Autodesk Inventor part; units mm, degrees
ref_plane "Work Plane1" through (-19.345, 0, 60) normal (1, 0, 0) x (0, 1, 0)
ref_plane "Work Plane2" through (-19.095, 0, 60) normal (1, 0, 0) x (0, 1, 0)
ref_plane "YZ Plane" through (0, 0, 0) normal (1, 0, 0) x (0, 1, 0)
sketch "Sketch1" plane through (0, 0, 0) normal (0, 0, 1) x (1, 0, 0)
  circle A0 centre (0, 0) radius 20
  dimension "d0" = 40
extrude "Extrusion1" add sketch "Sketch1" along normal blind 60
sketch "Sketch2" plane through (0, 0, 60) normal (0, 0, 1) x (1, 0, 0)
  circle A0 centre (0, 0) radius 20
  circle A1 centre (0, 0) radius 19.345
extrude "Extrusion2" add sketch "Sketch2" along normal blind 6.6 contours A1
sketch "Sketch3" plane through (0, 0, 66.6) normal (0, 0, 1) x (1, 0, 0)
  circle A0 centre (0, 0) radius 19.345
  circle A1 centre (0, 0) radius 20
  dimension "d5" = 40
extrude "Extrusion3" add sketch "Sketch3" along normal blind 38 contours A0 | A1
sketch "Sketch4" plane through (0, 0, 104.6) normal (0, 0, 1) x (1, 0, 0)
  circle A0 centre (0, 0) radius 20
  circle A1 centre (0, 0) radius 8
  dimension "d8" = 16
extrude "Extrusion4" add sketch "Sketch4" along normal blind 4 contours A1
sketch "Sketch5" plane through (0, 0, 108.6) normal (0, 0, 1) x (1, 0, 0)
  circle A0 centre (0, 0) radius 8
  line L0 (3.75, 2.9155) -> (3.75, -2.9155)
  line L1 (-3.75, -2.9155) -> (-3.75, 2.9155)
  arc A1 (-3.75, -2.9155) -> (3.75, -2.9155) centre (0, 0) ccw
  arc A2 (3.75, 2.9155) -> (-3.75, 2.9155) centre (0, 0) ccw
  point P0 (-3.75, 0)
  point P1 (0, 5.9024)
  dimension "d13" = 4.75
  dimension "d14" = 4.75
  dimension "d15" = 7.5
  dimension "d16" = 3.75
  dimension "d17" = 7.5
  dimension "d18" = 5.9024
extrude "Extrusion5" add sketch "Sketch5" along normal blind 14 contours L0 A1 L1 A2
sketch "Sketch6" plane through (0, 0, 122.6) normal (0, 0, 1) x (1, 0, 0)
  line L0 (3.75, 2.9155) -> (3.75, -2.9155)
  arc A0 (3.75, 2.9155) -> (-3.75, 2.9155) centre (0, 0) ccw
  line L1 (-3.75, -2.9155) -> (-3.75, 2.9155)
  arc A1 (-3.75, -2.9155) -> (3.75, -2.9155) centre (0, 0) ccw
  circle A2 centre (0, 0) radius 3.25
  dimension "d21" = 6.5
extrude "Extrusion6" add sketch "Sketch6" along normal blind 10 contours A2
chamfer "Chamfer1" distance 1 angle 45 1 edges at (-3.25, 0, 132.6)
chamfer "Chamfer2" distance 1 angle 80 1 edges at (-20, 0, 0) measured on face at (-2.364, 6.2334, 0)
ref_plane "Work Plane1" through (-19.345, 0, 60) normal (1, 0, 0) x (0, 1, 0)
ref_plane "Work Plane2" through (-19.095, 0, 60) normal (1, 0, 0) x (0, 1, 0)
sketch "Sketch8" plane through (-19.095, 0, 60) normal (1, 0, 0) x (0, 1, 0)
  circle A0 centre (0.0498, -2.6078) radius 0.75
  circle A1 centre (0, 4.3902) radius 0.75
  dimension "d31" = 1.5
  dimension "d32" = 1.5
extrude "Extrusion7" add sketch "Sketch8" against normal blind 10
sketch "Sketch9" plane through (0, 0, 104.6) normal (0, 0, 1) x (1, 0, 0)
  circle A0 centre (0, 0) radius 8
  circle A1 centre (0, 0) radius 20
  line L0 (-9, 9) -> (9, 9)
  line L1 (9, 9) -> (9, -9)
  line L2 (9, -9) -> (-9, -9)
  line L3 (-9, -9) -> (-9, 9)
  point P0 (0, 9)
  point P1 (-9, 0)
  dimension "d35" = 18
  dimension "d36" = 18
hole "Hole1" at (-9, 9, 104.6) at (9, 9, 104.6) at (9, -9, 104.6) at (-9, -9, 104.6) direction (0, 0, -1) diameter 2.487 depth 8 tip angle 118
equation "\"d32\" = d31"
equation "\"d36\" = d35"
properties part number "409A587"
Geometry check sheet. Reference: the model listing, model coordinates, mm. A direction names the side the tool comes from. Give positions to 0.01 mm unless a question says otherwise; leave off trailing zeros. Order: outer loops, then holes, each group sorted by start corner. A loop starts at its lowest first (then second) coordinate and runs counter-clockwise, first axis right, second up.
1. Sectioned sample at C-C (z = 33.5). Record the boundary of the cut face in (x, y).
Completed:
outline: circle Ø40 at (0, 0)
2. Sectioned sample at A-A (x = 0). Record the boundary of the cut face in (y, z) (3 decimals).
Completed:
outline: (-20, 5.671) - (-19, 0) - (19, 0) - (20, 5.671) - (20, 60) - (19.345, 60) - (19.345, 66.6) - (20, 66.6) - (20, 104.6) - (8, 104.6) - (8, 108.6) - (4.75, 108.6) - (4.75, 122.6) - (3.25, 122.6) - (3.25, 131.6) - (2.25, 132.6) - (-2.25, 132.6) - (-3.25, 131.6) - (-3.25, 122.6) - (-4.75, 122.6) - (-4.75, 108.6) - (-8, 108.6) - (-8, 104.6) - (-20, 104.6) - (-20, 66.6) - (-19.345, 66.6) - (-19.345, 60) - (-20, 60) - close
3. Depth check by flat-ended pin: pin 1 (1 mm diameter, centred on y = -4.5, z = 96, fed in from -X); pin 2 (1 mm diameter, centred on y = -15.5, z = 38.5, fed in from +X); pin 3 (12 mm diameter, centred on x = 7, y = -1, fed in from +Z); pin 4 (3 mm diameter, centred on x = 9, y = 9, fed in from +Z). Enter the tip coordinate at first touch or a pass-through.
Completed:
pin 1: stops at x = -19.6
pin 2: stops at x = 13.23
pin 3: stops at z = 132.6
pin 4: stops at z = 104.6
4. Access from +Z, -Z, +X, -X, +Y, -Y to the whole of each face (thin tool, end or side, straight path). Record for faces 1 (the face through (-2.579, 1.978, 127.037)), 2 (the face through (-8, 18, 60)), 3 (the face through (0.06, -4.75, 115.5)), 4 (the face through (-0.06, 4.75, 115.5)).
Completed:
face 1: +Z
face 2: none
face 3: +Z, -Y
face 4: +Z, +Y
5. Scan lines: line 1 (Y direction, x = -9, z = 99.5); line 2 (Z direction, x = 14.5, y = 10.5). Record each from-to range of solid material in increasing order.
Completed:
line 1: y = -17.86 to -10.24, -7.76 to 7.76, 10.24 to 17.86
line 2: z = 0 to 104.6
6. Sectioned sample at B-B (z = 112). Record the boundary of the cut face in (x, y), then the cut area to 3 significant figures.
Completed:
outline: (-3.75, -2.92) arc R4.75 ccw to (3.75, -2.92) - (3.75, 2.92) arc R4.75 ccw to (-3.75, 2.92) - close
area: 62.9 mm2
7. Draft check along X on faces 5 (the face through (-4.13, -18.61, 0.35)), 6 (the face through (9, 0, 104.6)), 7 (the face through (-9.84, 9.917, 100.544)). Enter one of: pulls with the +X half, pulls with the -X half, needs draft (parallel to the pull), parting line crosses it, or undercut.
Completed:
face 5: parting line crosses it
face 6: needs draft
face 7: undercut
